Source: CAD feature listing. Evaluate the final solid. Frame: model axes, mm. A direction names the side the tool comes from. Round coordinates to 2 decimals unless told otherwise and drop trailing zeros. Write each loop counter-clockwise with the first axis right and the second up, starting at its lowest first coordinate (ties: lowest second). Pieces come first, ordered by that corner, then holes.
from build123d import *

# Parameters (mm, degrees)
SALIENTE_EXTRUIR1_DEPTH    = 4.2
CROQUIS2_R                 = 6
SALIENTE_EXTRUIR2_DEPTH    = 12
CROQUIS3_R                 = 3
CORTAR_EXTRUIR1_DEPTH      = 19.627961062
CORTAR_EXTRUIR2_DEPTH      = 19.627961062
CORTAR_EXTRUIR2_DEPTH_BACK = 19.627961062
CROQUIS4_R                 = 2


with BuildPart() as part:
    # Croquis1 → Saliente-Extruir1 (new body)
    with BuildSketch(Plane(origin=(0, 0, 0), x_dir=(1, 0, 0), z_dir=(0, 1, 0))):
        Polygon((0, 6.951297241), (-6.02, 3.475648621), (-6.02, -3.475648621), (0, -6.951297241), (6.02, -3.475648621), (6.02, 3.475648621), align=None)
    extrude(amount=SALIENTE_EXTRUIR1_DEPTH)

    # Croquis2 → Saliente-Extruir2 (add)
    with BuildSketch(Plane(origin=(0, 4.2, 0), x_dir=(1, 0, 0), z_dir=(0, 1, 0))):
        with Locations(Location((0, 0, 0), (0, 0, 270))):
            Circle(CROQUIS2_R)
    extrude(amount=SALIENTE_EXTRUIR2_DEPTH)

    # Croquis3 → Cortar-Extruir1 (cut, through all)
    with BuildSketch(Plane(origin=(0, 16.2, 0), x_dir=(1, 0, 0), z_dir=(0, 1, 0))):
        with Locations(Location((0, 0, 0), (0, 0, 270))):
            Circle(CROQUIS3_R)
    extrude(amount=-CORTAR_EXTRUIR1_DEPTH, mode=Mode.SUBTRACT)

    # Croquis4 → Cortar-Extruir2 (cut, two sides: drawn at the far end of the back side and taken through both)
    with BuildSketch(Plane.XY.offset(-CORTAR_EXTRUIR2_DEPTH_BACK)):
        with Locations((0, 11.2)):
            Circle(CROQUIS4_R)
    extrude(amount=CORTAR_EXTRUIR2_DEPTH + CORTAR_EXTRUIR2_DEPTH_BACK, mode=Mode.SUBTRACT)


solid = part.part
1) Contact query for flat-ended pins moving along their axis: P1, Ø1.5, axis at x = -3, y = 11.5, coming from the +Z side; P2, Ø3.5, axis at x = 0, y = 11.2, coming from the +Z side; P3, Ø6, axis at x = -2, y = 12, coming from the +Z side; P4, Ø1, axis at y = 7, z = -1.5, coming from the -X side. Output: stop coordinate, or through.
Taken from the geometry:
P1: stops at z = 5.56
P2: passes through
P3: stops at z = 6
P4: stops at x = -5.92
2) Section query D-D on y = 11.5. Return the cut outline in (x, z).
Taken from the geometry:
outline: (-1.98, -5.66) - (-1.98, -2.26) arc R3 cw to (-1.98, 2.26) - (-1.98, 5.66) arc R6 ccw to start; (1.98, -5.66) arc R6 ccw to (1.98, 5.66) - (1.98, 2.26) arc R3 cw to (1.98, -2.26) - close
3) Material intervals for line 1 (Y direction, x = 0, z = 4.95); line 2 (X direction, y = 8, z = 0), sorted ascending.
Taken from the geometry:
line 1: y = 0 to 9.2, 13.2 to 16.2
line 2: x = -6 to -3, 3 to 6
4) Pull-direction query (X, two-part tool) for faces 3 (the face through (-3, 0, 1)), 4 (the face through (1.908, 11.801, -4.146)), 5 (the face through (6.02, 2, 0)), 6 (the face through (-2.968, 2.071, -5.238)); classes: released by +X, released by -X, zero draft, split by the parting line, or undercut.
Taken from the geometry:
face 3: zero draft
face 4: undercut
face 5: released by +X
face 6: released by -X
5) Section query B-B on y = 1. Return the cut outline in (x, z), then the cut area to 3 significant figures.
Taken from the geometry:
outline: (-6.02, -3.48) - (0, -6.95) - (6.02, -3.48) - (6.02, 3.48) - (0, 6.95) - (-6.02, 3.48) - close; hole circle Ø6 at (0, 0)
area: 97.3 mm2
6) Reachability of faces 1 (the face through (2.03, 8.21, -2.21)), 2 (the face through (-2.3, 10.12, 5.54)) from +Z, -Z, +X, -X, +Y, -Y: full face, straight path, thin tool, end or side. Return the list, or none.
Taken from the geometry:
face 1: +Y, -Y
face 2: +Y
